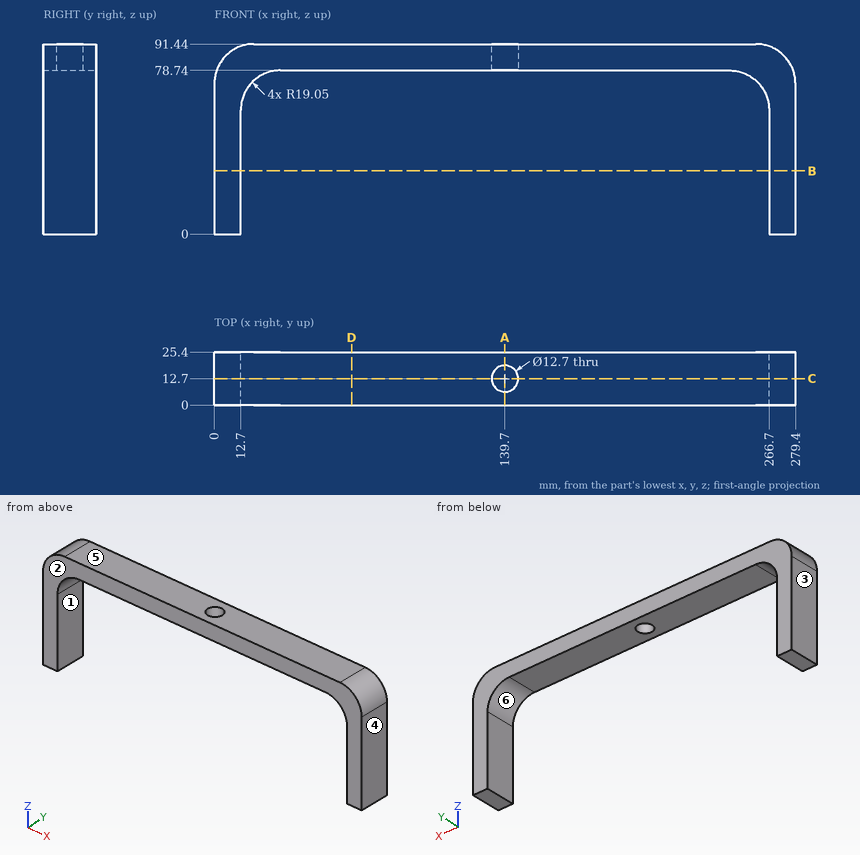
For this review, use the dimensioned drawing (mm, ordinates from the lowest corner) and the shaded views. A direction names the side the tool comes from. Give positions to 0.01 mm unless a question says otherwise; leave off trailing zeros. Order: outer loops, then holes, each group sorted by start corner. A loop starts at its lowest first (then second) coordinate and runs counter-clockwise, first axis right, second up. Notation, with made-up numbers: (-34.5, 63.5) - (5.5, 63.5) arc R15 cw to (5.5, 79.5) - close; hole circle Ø2 at (46.5, -31.5). An arc over 180 degrees is marked (long way). Use CSV: the item, a comma, the result in double quotes. Start each with the question number.
Q1. For line 1 (X direction, y = 12.5, z = 60.5); line 2 (Y direction, x = 139.7, z = 83.75); line 3 (Z direction, x = 56, y = 21.5), list the stretches that pass through material, from the lowest coordinate up.
Q2. Take a section at D-D (x = 66). State the section outline as (y, z) points, and give its area (3 significant figures).
Q3. Machinability: for the marked faces 5 and 6, which of the approach directions +Z, -Z, +X, -X, +Y, -Y give a long, thin tool a straight path to every point of the face, cutting with its end or side? Answer none if there is none.
Q4. Take a section at C-C (y = 12.7). State the section outline as (x, z) points.
Q5. For P1, Ø7.5, axis at x = 121.5, y = 13, coming from the -Z side; P2, Ø10, axis at y = 21.5, z = 28.5, coming from the -X side, all flat-tipped, find the tip position at first contact; note any pin that passes through.
Q6. Draft analysis for pull direction X (two halves, no side actions). For the marked faces 1, 2, 3 and 4, state which applies: pulls with the +X half, pulls with the -X half, needs draft (parallel to the pull), parting line crosses it, or undercut.
Q7. Take a section at A-A (x = 139.7). State the section outline as (y, z) points.
Q8. Take a section at B-B (z = 30.5). State the section outline as (x, y) points, and give its area (3 significant figures).
Calculated:
1,line 1,"x = 0 to 12.72, 266.68 to 279.4"
1,line 2,"y = 0 to 6.35, 19.05 to 25.4"
1,line 3,"z = 78.74 to 91.44"
2,outline,"(0, 78.74) - (25.4, 78.74) - (25.4, 91.44) - (0, 91.44) - close"
2,area,"323 mm²"
3,face 5,"+Z, +X, -X, +Y, -Y"
3,face 6,"-Z, +Y, -Y"
4,outline,"(0, 0) - (12.7, 0) - (12.7, 59.69) arc R19.05 cw to (31.75, 78.74) - (133.35, 78.74) - (133.35, 91.44) - (19.05, 91.44) arc R19.05 ccw to (0, 72.39) - close; (146.05, 78.74) - (247.65, 78.74) arc R19.05 cw to (266.7, 59.69) - (266.7, 0) - (279.4, 0) - (279.4, 72.39) arc R19.05 ccw to (260.35, 91.44) - (146.05, 91.44) - close"
5,P1,"stops at z = 78.74"
5,P2,"stops at x = 0"
6,face 1,"undercut"
6,face 2,"needs draft"
6,face 3,"pulls with the -X half"
6,face 4,"pulls with the +X half"
7,outline,"(0, 78.74) - (6.35, 78.74) - (6.35, 91.44) - (0, 91.44) - close; (19.05, 78.74) - (25.4, 78.74) - (25.4, 91.44) - (19.05, 91.44) - close"
8,outline,"(0, 0) - (12.7, 0) - (12.7, 25.4) - (0, 25.4) - close; (266.7, 0) - (279.4, 0) - (279.4, 25.4) - (266.7, 25.4) - close"
8,area,"645 mm²"
